from build123d import *

# Parameters (mm, degrees)
SKETCH6_R           = 1
SKETCH6_R_2         = 3.5
BOSS_EXTRUDE2_DEPTH = 3.5
FILLET1_R           = 1.5


with BuildPart() as part:
    # Sketch6 → Boss-Extrude2 (new body)
    with BuildSketch(Plane.XY):
        with BuildLine():
            Line((-18.481457554, 7.854026145), (-4.341757745, -4.837265724))
            ThreePointArc((-4.341757745, -4.837265724), (4.866357239, -4.309126039), (4.276299413, 4.895228629))
            Line((4.276299413, 4.895228629), (-9.968273897, 17.338786449))
            Line((-9.968273897, 17.338786449), (-7.460072509, 20.133239137))
            Line((-7.460072509, 20.133239137), (-53.070551784, 61.07158384))
            Line((-53.070551784, 61.07158384), (-93.636038969, 20.506096654))
            Line((-93.636038969, 20.506096654), (-91.161165235, 18.03122292))
            Line((-91.161165235, 18.03122292), (-104.596194078, 4.596194078))
            ThreePointArc((-104.596194078, 4.596194078), (-104.596194078, -4.596194078), (-95.403805922, -4.596194078))
            Line((-95.403805922, -4.596194078), (-81.96877708, 8.838834765))
            Line((-81.96877708, 8.838834765), (-79.493903346, 6.363961031))
            Line((-79.493903346, 6.363961031), (-52.327712868, 33.530151508))
            Line((-52.327712868, 33.530151508), (-20.819327109, 5.249344602))
            Line((-20.819327109, 5.249344602), (-18.481457554, 7.854026145))
        make_face()
        with Locations((-52.699132326, 47.300867674)):
            Circle(SKETCH6_R, mode=Mode.SUBTRACT)
        Circle(SKETCH6_R_2, mode=Mode.SUBTRACT)
        with Locations((-100, 0)):
            Circle(SKETCH6_R_2, mode=Mode.SUBTRACT)
        with Locations((-86.564971157, 20.506096654)):
            Circle(SKETCH6_R, mode=Mode.SUBTRACT)
        with Locations((-15.26505452, 20.420041883)):
            Circle(SKETCH6_R, mode=Mode.SUBTRACT)
        with Locations((-21.944681819, 12.978094615)):
            Circle(SKETCH6_R, mode=Mode.SUBTRACT)
        with Locations((-79.493903346, 13.435028843)):
            Circle(SKETCH6_R, mode=Mode.SUBTRACT)
    extrude(amount=BOSS_EXTRUDE2_DEPTH)

    # Fillet1
    fillet1_edges = [part.edges().sort_by_distance(p)[0] for p in [
        (-91.161165235, 18.03122292, 1.75),
        (-93.636038969, 20.506096654, 1.75),
        (-53.070551784, 61.07158384, 1.75),
        (-7.460072509, 20.133239137, 1.75),
        (-9.968273897, 17.338786449, 1.75),
    ]]
    fillet(fillet1_edges, radius=FILLET1_R)


solid = part.part
Design review of the part built by this model. Coordinates are the model's own, in mm. A direction names the side the tool comes from. Give positions to 0.01 mm unless a question says otherwise; leave off trailing zeros. Loops run counter-clockwise (first coordinate to the right, second up) from the corner with the lowest first, then second, coordinate; pieces in that order, holes last. Notation, with made-up numbers: (76.5, 10.25) - (134.5, 10.25) arc R12 ccw to (134.5, 23.25) - close; hole circle Ø10 at (-5, 41). An arc over 180 degrees is marked (long way). Use CSV: the item, a comma, the result in double quotes. Start each with the question number.
1. Add section A-A (x = 0). State the section outline as (y, z) points, plus the area to 3 significant figures.
2. Wall thickness on L1, parallel to X at y = 2, z = 1.6; L2, parallel to X at y = 7, z = 0.85; L3, parallel to X at y = 5, z = 0.4: over which ranges is each line inside the solid? List them lowest first.
3. Machinability: for faces 5 (the cylindrical face through (-104.7, -4.49, 1.73)), 6 (the flat face through (-19.67, 6.53, 1.73)), which of the approach directions +Z, -Z, +X, -X, +Y, -Y give a long, thin tool a straight path to every point of the face, cutting with its end or side? Answer none if there is none.
4. Add section B-B (y = 0). State the section outline as (x, z) points.
5. Add section D-D (x = -77). State the section outline as (y, z) points, plus the area to 3 significant figures.
6. Add section C-C (x = -100). State the section outline as (y, z) points, plus the area to 3 significant figures.
7. Draft analysis for pull direction Y (two halves, no side actions). For faces 1 (the cylindrical face through (-86.695, 21.498, 1.726)), 2 (the cylindrical face through (-22.682, 13.654, 1.726)), 3 (the flat face through (-46, 32, 3.5)), 4 (the cylindrical face through (4.77, -4.416, 1.726)), state which applies: released by +Y, released by -Y, zero draft, split by the parting line, or undercut.
8. Insertion check: P1, Ø3, axis at x = -76.5, y = 27.5, coming from the -Z side; P2, Ø1, axis at x = -74, z = 0.5, coming from the +Y side; P3, Ø2, axis at y = 9, z = 2, coming from the +X side. Each pin has a flat end and moves straight along its axis. Give the tip position at first contact, or say it passes through.
Results found:
1,outline,"(-6.5, 0) - (-3.5, 0) - (-3.5, 3.5) - (-6.5, 3.5) - close; (3.5, 0) - (8.63, 0) - (8.63, 3.5) - (3.5, 3.5) - close"
1,area,"28.5 mm²"
2,L1,"x = -106.18 to -102.87, -97.13 to -88.81, -11.96 to -2.87, 2.87 to 6.18"
2,L2,"x = -102.19 to -83.81, -80.13 to -78.86, -22.77 to -19.25, -17.53 to 1.87"
2,L3,"x = -104.19 to -85.81, -15.3 to 4.16"
3,face 5,"+Z, -Z"
3,face 6,"+Z, -Z, -Y"
4,outline,"(-106.5, 0) - (-103.5, 0) - (-103.5, 3.5) - (-106.5, 3.5) - close; (-96.5, 0) - (-90.81, 0) - (-90.81, 3.5) - (-96.5, 3.5) - close; (-9.73, 0) - (-3.5, 0) - (-3.5, 3.5) - (-9.73, 3.5) - close; (3.5, 0) - (6.5, 0) - (6.5, 3.5) - (3.5, 3.5) - close"
5,outline,"(8.86, 0) - (37.14, 0) - (37.14, 3.5) - (8.86, 3.5) - close"
5,area,"99.0 mm²"
6,outline,"(-6.5, 0) - (-3.5, 0) - (-3.5, 3.5) - (-6.5, 3.5) - close; (3.5, 0) - (9.19, 0) - (9.19, 3.5) - (3.5, 3.5) - close"
6,area,"30.4 mm²"
7,face 1,"undercut"
7,face 2,"undercut"
7,face 3,"zero draft"
7,face 4,"split by the parting line"
8,P1,"stops at z = 0"
8,P2,"stops at y = 40.64"
8,P3,"stops at x = 0.72"
